```python
from build123d import *

# Parameters (mm, degrees)
SKETCH_2_R             = 40
EXTRUDE_1_DEPTH        = 3
SKETCH_3_R             = 43
SKETCH_3_R_2           = 1.5
SKETCH_3_R_3           = 1.75
EXTRUDE_2_DEPTH        = 2
SKETCH_4_R             = 1.7
EXTRUDE_3_DEPTH        = 6
SKETCH_6_W             = 19.489388493
SKETCH_6_H             = 55
EXTRUDE_4_DEPTH        = 9.662698808
SKETCH_7_W             = 5
SKETCH_7_H             = 7.2
EXTRUDE_5_DEPTH        = 20
FILLET_1_R             = 5
SKETCH_8_R             = 1.75
CUT_EXTRUDE_1_DEPTH    = 8
FILLET_1_OF_MIRROR_1_R = 5
FILLET_2_R             = 5
SKETCH_10_R            = 5
SKETCH_10_R_2          = 1.7
EXTRUDE_6_DEPTH        = 4
EXTRUDE_7_DEPTH        = 15.489388493
SKETCH_13_W            = 48.978361992
SKETCH_13_H            = 5.952940671
EXTRUDE_8_DEPTH        = 2


with BuildPart() as part:
    # 草图2 → 凸台-拉伸1 (new body)
    with BuildSketch(Plane.XY):
        Circle(SKETCH_2_R)
        with BuildLine():
            Line((-3.843778342, 6.657619381), (-10.418112816, 9.210167583))
            ThreePointArc((-10.418112816, 9.210167583), (-13.856406461, 8), (-13.185295508, 4.417266567))
            Line((-13.185295508, 4.417266567), (-7.687556684, 0))
            Line((-7.687556684, 0), (-13.185295508, -4.417266567))
            ThreePointArc((-13.185295508, -4.417266567), (-13.856406461, -8), (-10.418112816, -9.210167583))
            Line((-10.418112816, -9.210167583), (-3.843778342, -6.657619381))
            Line((-3.843778342, -6.657619381), (-2.767182691, -13.62743415))
            ThreePointArc((-2.767182691, -13.62743415), (0, -16), (2.767182691, -13.62743415))
            Line((2.767182691, -13.62743415), (3.843778342, -6.657619381))
            Line((3.843778342, -6.657619381), (10.418112816, -9.210167583))
            ThreePointArc((10.418112816, -9.210167583), (13.856406461, -8), (13.185295508, -4.417266567))
            Line((13.185295508, -4.417266567), (7.687556684, 0))
            Line((7.687556684, 0), (13.185295508, 4.417266567))
            ThreePointArc((13.185295508, 4.417266567), (13.856406461, 8), (10.418112816, 9.210167583))
            Line((10.418112816, 9.210167583), (3.843778342, 6.657619381))
            Line((3.843778342, 6.657619381), (2.767182691, 13.62743415))
            ThreePointArc((2.767182691, 13.62743415), (0, 16), (-2.767182691, 13.62743415))
            Line((-2.767182691, 13.62743415), (-3.843778342, 6.657619381))
        make_face(mode=Mode.SUBTRACT)
    extrude(amount=-EXTRUDE_1_DEPTH)

    # 草图3 → 凸台-拉伸2 (add)
    with BuildSketch(Plane.XY):
        Circle(SKETCH_3_R)
        with Locations((0, -7.5)):
            Circle(SKETCH_3_R_2, mode=Mode.SUBTRACT)
        with Locations((-6.495190528, -3.75)):
            Circle(SKETCH_3_R_2, mode=Mode.SUBTRACT)
        with Locations((-6.495190528, 3.75)):
            Circle(SKETCH_3_R_2, mode=Mode.SUBTRACT)
        with Locations((0, 7.5)):
            Circle(SKETCH_3_R_2, mode=Mode.SUBTRACT)
        with Locations((6.495190528, 3.75)):
            Circle(SKETCH_3_R_2, mode=Mode.SUBTRACT)
        with Locations((6.495190528, -3.75)):
            Circle(SKETCH_3_R_2, mode=Mode.SUBTRACT)
        Circle(SKETCH_3_R_3, mode=Mode.SUBTRACT)
    extrude(amount=EXTRUDE_2_DEPTH)

    # 草图4 → 凸台-拉伸3 (add, symmetric)
    with BuildSketch(Plane(origin=(0, 0, 0), x_dir=(0, 0, -1), z_dir=(1, 0, 0))):
        with BuildLine():
            Line((-21.791018214, 17.858318105), (-2, 11))
            Line((-2, 11), (-2, 37))
            Line((-2, 37), (-21.791018214, 30.141681895))
            ThreePointArc((-21.791018214, 30.141681895), (-26.162698808, 24), (-21.791018214, 17.858318105))
        make_face()
        with Locations((-19.662698808, 24)):
            Circle(SKETCH_4_R, mode=Mode.SUBTRACT)
    extrude(amount=EXTRUDE_3_DEPTH, both=True)

    # 草图6 → 凸台-拉伸4 (add)
    with BuildSketch(Plane(origin=(0, 0, 0), x_dir=(-1, 0, 0), z_dir=(0, 0, -1))):
        with Locations((33.255305753, 13.65)):
            Rectangle(SKETCH_6_W, SKETCH_6_H)
    extrude_4 = extrude(amount=-EXTRUDE_4_DEPTH)

    # 草图7 → 凸台-拉伸5 (add)
    with BuildSketch(Plane.XY.offset(9.662698808)):
        with Locations((-36.510611507, 37.55)):
            Rectangle(SKETCH_7_W, SKETCH_7_H)
        with Locations((-36.510611507, -10.25)):
            Rectangle(SKETCH_7_W, SKETCH_7_H)
    extrude_5 = extrude(amount=EXTRUDE_5_DEPTH)

    # 圆角1
    # the kernel refuses this fillet: 5 mm, written as the material it adds along each edge
    with BuildSketch(Plane(origin=(-39.010611507, -13.85, 9.662698808), x_dir=(-1.0, 0, 9.057736173164017e-11), z_dir=(0, 1, 0)), Plane(origin=(-39.010611507, 33.95, 9.662698808), x_dir=(-1.0, 0, 9.057736173164017e-11), z_dir=(0, 1, 0))) as fillet_1_piece_1:
        with BuildLine():
            CenterArc((5, 4.896801444), FILLET_1_R, 179.999999995, 78.338907052)
            Line((0, 4.896801444), (-0.1, 4.896801444))
            Line((-0.1, 4.896801444), (-0.1, 0))
            Line((-0.1, 0), (0, -0.1))
            ThreePointArc((0, -0.1), (1.994694247, -0.1), (3.969176263, -0.097936029))
            Line((3.969176263, -0.097936029), (3.989388493, 0))
        make_face()
    extrude(amount=7.2)

    # 草图8 → 切除-拉伸1 (cut)
    with BuildSketch(Plane(origin=(-34.010611507, 0, 0), x_dir=(0, 0, -1), z_dir=(1, 0, 0))):
        with Locations((-14.662698808, 37.965)):
            Circle(SKETCH_8_R)
        with Locations((-24.662698808, 37.965)):
            Circle(SKETCH_8_R)
        with Locations((-14.662698808, -10.665)):
            Circle(SKETCH_8_R)
        with Locations((24.662698808, -10.665)):
            Circle(SKETCH_8_R)
    cut_extrude_1 = extrude(amount=-CUT_EXTRUDE_1_DEPTH, mode=Mode.SUBTRACT)

    # 镜向1: 凸台-拉伸4, 凸台-拉伸5, 切除-拉伸1 across plane
    add(extrude_4.mirror(Plane(origin=(0, 0, 0), x_dir=(0, 0, 1), z_dir=(1, 0, 0))))
    add(extrude_5.mirror(Plane(origin=(0, 0, 0), x_dir=(0, 0, 1), z_dir=(1, 0, 0))))
    add(cut_extrude_1.mirror(Plane(origin=(0, 0, 0), x_dir=(0, 0, 1), z_dir=(1, 0, 0))), mode=Mode.SUBTRACT)

    # 圆角1 of 镜向1
    # the kernel refuses this fillet: 5 mm, written as the material it adds along each edge
    with BuildSketch(Plane(origin=(39.010611507, -13.85, 9.662698808), x_dir=(1.0, 0, 9.057736173164017e-11), z_dir=(0, 1, 0))) as fillet_1_of_mirror_1_piece_1_section:
        with BuildLine():
            CenterArc((5, -4.896801444), FILLET_1_OF_MIRROR_1_R, 101.661092954, 78.338907052)
            Line((0, -4.896801444), (-0.1, -4.896801444))
            Line((-0.1, -4.896801444), (-0.1, 0))
            Line((-0.1, 0), (0, 0.1))
            ThreePointArc((0, 0.1), (1.994694247, 0.1), (3.969176263, 0.097936029))
            Line((3.969176263, 0.097936029), (3.989388493, 0))
        make_face()
    fillet_1_of_mirror_1_piece_1 = extrude(amount=7.2, mode=Mode.PRIVATE)
    fillet_1_of_mirror_1_piece_1 = fillet_1_of_mirror_1_piece_1 - Plane(origin=(40.024571276, -10.665, 14.662698808), x_dir=(0, 0, -1), z_dir=(-1, 0, 0)) * Cylinder(1.75, 34, mode=Mode.PRIVATE)
    add(fillet_1_of_mirror_1_piece_1)
    with BuildSketch(Plane(origin=(39.010611507, 33.95, 9.662698808), x_dir=(1.0, 0, 9.057736173164017e-11), z_dir=(0, 1, 0))) as fillet_1_of_mirror_1_piece_2_section:
        with BuildLine():
            CenterArc((5, -4.896801444), FILLET_1_OF_MIRROR_1_R, 101.661092954, 78.338907052)
            Line((0, -4.896801444), (-0.1, -4.896801444))
            Line((-0.1, -4.896801444), (-0.1, 0))
            Line((-0.1, 0), (0, 0.1))
            ThreePointArc((0, 0.1), (1.994694247, 0.1), (3.969176263, 0.097936029))
            Line((3.969176263, 0.097936029), (3.989388493, 0))
        make_face()
    fillet_1_of_mirror_1_piece_2 = extrude(amount=7.2, mode=Mode.PRIVATE)
    fillet_1_of_mirror_1_piece_2 = fillet_1_of_mirror_1_piece_2 - Plane(origin=(40.024571271, 37.965, 14.662698808), x_dir=(0, 0, -1), z_dir=(-1, 0, 0)) * Cylinder(1.75, 34, mode=Mode.PRIVATE)
    add(fillet_1_of_mirror_1_piece_2)

    # 圆角2
    # the kernel refuses this fillet: 5 mm, written as the material it adds along each edge
    with BuildSketch(Plane(origin=(-6, 11, 2), x_dir=(0, -1, 0), z_dir=(1, 0, 0))) as fillet_2_piece_1_section:
        with BuildLine():
            CenterArc((FILLET_2_R * 0.711805115944, -FILLET_2_R), FILLET_2_R, 90, 70.886911337)
            Line((-FILLET_2_R * 0.233069021814, -FILLET_2_R * 0.672566245179), (0, 0))
            Line((0, 0), (FILLET_2_R * 0.711805115944, 0))
        make_face()
    fillet_2_piece_1 = extrude(amount=12, mode=Mode.PRIVATE)
    fillet_2_piece_1 = fillet_2_piece_1 - Plane(origin=(0, 7.5, 2.750651106), x_dir=(1, 0, 0), z_dir=(0, 0, -1)) * Cylinder(1.5, 39, mode=Mode.PRIVATE)
    add(fillet_2_piece_1)
    with BuildSketch(Plane(origin=(-6, 37, 2), x_dir=(0, 1, 0), z_dir=(1, 0, 0))) as fillet_2_piece_2:
        with BuildLine():
            CenterArc((FILLET_2_R * 0.711805115944, FILLET_2_R), FILLET_2_R, 199.113088663, 70.886911337)
            Line((-FILLET_2_R * 0.233069021814, FILLET_2_R * 0.672566245179), (0, 0))
            Line((0, 0), (FILLET_2_R * 0.711805115944, 0))
        make_face()
    extrude(amount=12)

    # 草图10 → 凸台-拉伸6 (add)
    # profile 1 of 2: a face of its own
    with BuildSketch(Plane(origin=(-23.510611507, 0, 0), x_dir=(0, 0, -1), z_dir=(1, 0, 0))):
        with BuildLine():
            Line((0, 41.15), (-56.313238783, 60.858696746))
            ThreePointArc((-56.313238783, 60.858696746), (-53.887028683, 59.032613027), (-52.964920964, 56.139380484))
            ThreePointArc((-52.964920964, 56.139380484), (-55.468901732, 51.806957606), (-60.472876161, 51.813856154))
            Line((-60.472876161, 51.813856154), (-29.662698808, 33.95))
            Line((-29.662698808, 33.95), (-9.662698808, 33.95))
            Line((-9.662698808, 33.95), (-9.662698808, 41.15))
            Line((-9.662698808, 41.15), (0, 41.15))
        make_face()
    # profile 2 of 2: a face of its own
    with BuildSketch(Plane(origin=(-23.510611507, 0, 0), x_dir=(0, 0, -1), z_dir=(1, 0, 0))):
        with Locations((-57.964920964, 56.139380484)):
            Circle(SKETCH_10_R)
        with Locations((-57.964920964, 56.139380484)):
            Circle(SKETCH_10_R_2, mode=Mode.SUBTRACT)
    extrude(amount=-EXTRUDE_6_DEPTH)

    # 草图11 → 凸台-拉伸7 (add)
    with BuildSketch(Plane.ZY.offset(43)):
        Polygon((0, 41.15), (29.662698808, 41.15), (29.662698808, 46.138093671), (14.25237364, 46.138093671), align=None)
    extrude(amount=-EXTRUDE_7_DEPTH)

    # 草图13 → 凸台-拉伸8 (add)
    with BuildSketch(Plane(origin=(0, 0, 0), x_dir=(-1, 0, 0), z_dir=(0, 0, -1))):
        with Locations((-0.978569489, 38.173529665)):
            Rectangle(SKETCH_13_W, SKETCH_13_H)
    extrude(amount=-EXTRUDE_8_DEPTH)


solid = part.part
```
The model under review builds one solid part; all positions refer to its coordinate system, in mm. A direction names the side the tool comes from. Give positions to 0.01 mm unless a question says otherwise; leave off trailing zeros. Write each loop counter-clockwise with the first axis right and the second up, starting at its lowest first coordinate (ties: lowest second). Pieces come first, ordered by that corner, then holes.
(1) Consider section D-D, the plane x = 30.5. Give the boundary of the cut face in (y, z), and give its area (3 significant figures).
(2) For P1, Ø4.5, axis at x = 0, y = 0, coming from the -Z side; P2, Ø6, axis at x = -35.5, y = 40, coming from the +Z side; P3, Ø4.5, axis at x = 38, z = 24, coming from the -Y side, all flat-tipped, find the tip position at first contact; note any pin that passes through.
(3) Consider section C-C, the plane z = 7.5. Give the boundary of the cut face in (x, y).
(4) To check wall thickness, follow L1, parallel to X at y = 0, z = 9.5; L2, parallel to Y at x = -38, z = 21; L3, parallel to Z at x = -2, y = -26.5. State the ranges of each line that lie inside material, in increasing order.
(5) The part is to be moulded in two halves that separate along X. For faces 4 (the cylindrical face through (40.165, 37.5, 11.364)), 5 (the flat face through (3, 0, 0)), 6 (the cylindrical face through (-5.1, 3.2, 1)), 7 (the cylindrical face through (-36.61, -11.34, 13.05)), say which applies: released by +X, released by -X, zero draft, split by the parting line, or undercut.
(6) Tool access review of faces 1 (the flat face through (23.511, 13, 6)), 2 (the cylindrical face through (-36.61, 39.44, 13.72)), 3 (the cylindrical face through (-8.67, -39.05, -1.48)): name each direction out of +Z, -Z, +X, -X, +Y, -Y from which nothing blocks a thin tool from reaching the whole face with its end or side.
(7) Consider section B-B, the plane y = 24. Give the boundary of the cut face in (x, z).
(8) Consider section A-A, the plane x = 0. Give the number of separate pieces and of enclosed holes in the cut face, and give its area (3 significant figures).
Returned:
1. outline: (-30.31, 0) - (-25.88, 0) - (-25.88, -3) - (25.88, -3) - (25.88, 0) - (41.15, 0) - (41.15, 9.66) - (-13.85, 9.66) - (-13.85, 2) - (-30.31, 2) - close
1. area: 720 mm2
2. P1: stops at z = 0
2. P2: stops at z = 29.66
2. P3: stops at y = -13.85
3. outline: (-43, -13.85) - (-23.51, -13.85) - (-23.51, 43.77) - (-43, 43.77) - close; (-6, 12.91) - (6, 12.91) - (6, 35.09) - (-6, 35.09) - close; (23.51, -13.85) - (43, -13.85) - (43, 41.15) - (23.51, 41.15) - close
4. L1: x = -43 to -23.51, 23.51 to 43
4. L2: y = -13.85 to -6.65, 33.95 to 46.14
4. L3: z = -3 to 2
5. face 4: released by +X
5. face 5: undercut
5. face 6: undercut
5. face 7: zero draft
6. face 1: +Z, +Y, -Y
6. face 2: -X
6. face 3: -Z
7. outline: (-43, 0) - (-32, 0) - (-32, -3) - (32, -3) - (32, 0) - (43, 0) - (43, 9.66) - (23.51, 9.66) - (23.51, 2) - (6, 2) - (6, 17.96) - (-6, 17.96) - (-6, 2) - (-23.51, 2) - (-23.51, 9.66) - (-43, 9.66) - close; (-6, 21.36) - (6, 21.36) - (6, 26.16) - (-6, 26.16) - close
8. separate pieces: 4
8. enclosed holes: 1
8. area: 710 mm2
